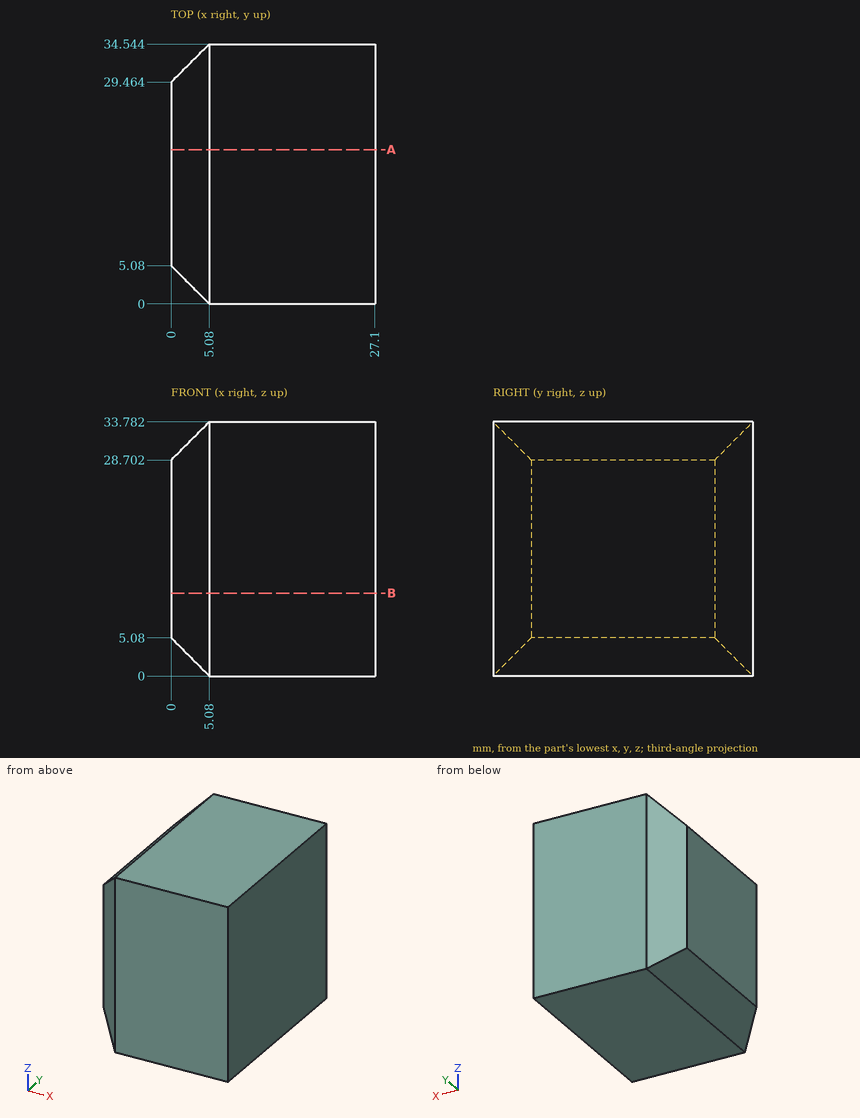
Geometry check sheet. Reference: drawing and pictorial views, mm from the part's lowest x, y, z. Give positions to 0.01 mm unless a question says otherwise; leave off trailing zeros. Order: outer loops, then holes, each group sorted by start corner. A loop starts at its lowest first (then second) coordinate and runs counter-clockwise, first axis right, second up. Notation, with made-up numbers: (38, 27.25) - (66, 27.25) arc R9 cw to (66, 32.25) - close; hole circle Ø8 at (39.5, 39). An arc over 180 degrees is marked (long way). Answer as CSV lines item,"result". Start each with the question number.
Item 1: Material ranges on L1, parallel to X at y = 7, z = 29; L2, parallel to Y at x = 5, z = 14; L3, parallel to Z at x = 2, y = 22.5, recorded low to high.
Item 2: Section check B-B, the plane z = 11. Record the boundary of the cut face in (x, y).
Item 3: Section check A-A, the plane y = 20.5. Record the boundary of the cut face in (x, z).
Filled in:
1,L1,"0.3 to 27.1"
1,L2,"0.08 to 34.46"
1,L3,"3.08 to 30.7"
2,outline,"(0, 5.08) - (5.08, 0) - (27.1, 0) - (27.1, 34.54) - (5.08, 34.54) - (0, 29.46) - close"
3,outline,"(0, 5.08) - (5.08, 0) - (27.1, 0) - (27.1, 33.78) - (5.08, 33.78) - (0, 28.7) - close"
